Read the model definition and answer for the solid it produces. Units are mm, in the model's axes. Face numbers are marked on the shaded views. A direction names the side the tool comes from. Round coordinates to 2 decimals unless told otherwise and drop trailing zeros. Order: outer loops, then holes, each group sorted by start corner. A loop starts at its lowest first (then second) coordinate and runs counter-clockwise, first axis right, second up. Notation, with made-up numbers: (41.5, 79) -> (81.5, 79) arc R21 cw to (81.5, 109) -> close; hole circle Ø6 at (33.5, -37). An arc over 180 degrees is marked (long way). Answer as a JSON object with one key per item and string values. Group by question number.
Item 1: The mould has two halves that part along Z. Classify the marked faces 1, 2, 3 and 4: pulls with the +Z half, pulls with the -Z half, needs draft (parallel to the pull), parting line crosses it, or undercut.
Item 2: Section D-D, the plane z = 30 is taken. Write down the section's boundary in (x, y).
Item 3: Section A-A, the plane z = 5.5 is taken. Write down the section's boundary in (x, y), plus the area to 3 significant figures.
Item 4: For the marked faces 5 and 6, determine the directions among +Z, -Z, +X, -X, +Y, -Y from which every point of the face is accessible in a straight line to the end or side of a thin tool.
Item 5: Given P1, Ø9, axis at x = -70, y = 5, coming from the +Z side; P2, Ø17, axis at x = -71.95, y = 0, coming from the -Z side; P3, Ø4, axis at y = -5, z = 26, coming from the +X side, each flat-ended and moving along its own axis, determine where each tip first touches the part or whether it passes through.
Item 6: Section C-C, the plane y = 4.25 is taken. Write down the section's boundary in (x, z).
Item 7: Section B-B, the plane x = 130 is taken. Write down the section's boundary in (y, z), plus the area to 3 significant figures.
Item 8: Consider probe 1 along X at (y, z) = (-1.5, -14.5); probe 2 along X at (y, z) = (-1.25, 15); probe 3 along X at (y, z) = (-8.75, -20.5). Determine where each line is inside the solid, lowest interval first. Write a range as from..to.
from build123d import *
from build123d.topology import SkipClean

# Parameters (mm, degrees)
SKETCH1_R           = 50
BOSS_EXTRUDE4_DEPTH = 10
SKETCH4_R           = 50
BOSS_EXTRUDE5_DEPTH = 5
BOSS_EXTRUDE6_START = 5
SKETCH5_R           = 50
BOSS_EXTRUDE6_DEPTH = 5
SKETCH9_R           = 15
SKETCH9_R_2         = 7.5
BOSS_EXTRUDE8_DEPTH = 40
CUT_EXTRUDE1_START  = 50
SKETCH11_R          = 15
CUT_EXTRUDE1_DEPTH  = 50
BOSS_EXTRUDE9_START = 12
SKETCH12_R          = 7.5
BOSS_EXTRUDE9_DEPTH = 12


with BuildPart() as part:
    # Sketch1 → Boss-Extrude4 (new, symmetric)
    # profile 1 of 2: a face of its own
    with BuildSketch(Plane(origin=(0, 0, 0), x_dir=(1, 0, 0), z_dir=(0, 1, 0))):
        with BuildLine():
            Line((109.631487436, 59.370873009), (-60.952961118, 36.317806))
            Line((-60.952961118, 36.317806), (-60.952961118, -47.492515538))
            Line((-60.952961118, -47.492515538), (113.395395748, -59.936377162))
            ThreePointArc((113.395395748, -59.936377162), (57.696778774, -1.980561591), (109.631487436, 59.370873009))
        make_face()
        with BuildLine():
            Line((-46.622582391, 28.163534109), (48.543183, 41.024394434))
            ThreePointArc((48.543183, 41.024394434), (53.334657365, 38.899688702), (53.596610708, 33.664807473))
            ThreePointArc((53.596610708, 33.664807473), (45.011329084, -2.407953952), (56.056582269, -37.805038006))
            ThreePointArc((56.056582269, -37.805038006), (56.147884391, -43.057885165), (51.492525841, -45.492710855))
            Line((51.492525841, -45.492710855), (-46.308923365, -38.512273973))
            ThreePointArc((-46.308923365, -38.512273973), (-49.612183114, -36.932319839), (-50.952961118, -33.524960981))
            Line((-50.952961118, -33.524960981), (-50.952961118, 23.208576253))
            ThreePointArc((-50.952961118, 23.208576253), (-49.717805495, 26.498856913), (-46.622582391, 28.163534109))
        make_face(mode=Mode.SUBTRACT)
    # profile 2 of 2: a face of its own
    with BuildSketch(Plane(origin=(0, 0, 0), x_dir=(1, 0, 0), z_dir=(0, 1, 0))):
        with BuildLine():
            ThreePointArc((177.666942704, -0.088621259), (157.15031062, 45.089511261), (109.631487436, 59.370873009))
            ThreePointArc((109.631487436, 59.370873009), (57.696778774, -1.980561591), (113.395395748, -59.936377162))
            ThreePointArc((113.395395748, -59.936377162), (158.555248995, -43.999285211), (177.666942704, -0.088621259))
        make_face()
        with Locations(Location((117.666942704, -0.088621259, 0), (0, 0, 270))):
            Circle(SKETCH1_R, mode=Mode.SUBTRACT)
    extrude(amount=BOSS_EXTRUDE4_DEPTH, both=True)

    # Sketch4 → Boss-Extrude5 (add)
    with BuildSketch(Plane(origin=(0, 10, 0), x_dir=(1, 0, 0), z_dir=(0, 1, 0))):
        with BuildLine():
            ThreePointArc((109.631487436, 59.370873009), (57.696778774, -1.980561591), (113.395395748, -59.936377162))
            ThreePointArc((113.395395748, -59.936377162), (158.555248995, -43.999285211), (177.666942704, -0.088621259))
            ThreePointArc((177.666942704, -0.088621259), (157.15031062, 45.089511261), (109.631487436, 59.370873009))
        make_face()
        with Locations(Location((117.666942704, -0.088621259, 0), (0, 0, 270))):
            Circle(SKETCH4_R, mode=Mode.SUBTRACT)
    extrude(amount=BOSS_EXTRUDE5_DEPTH)

    # Sketch5 → Boss-Extrude6 (add)
    with BuildSketch(Plane.XZ.offset(10).offset(BOSS_EXTRUDE6_START)):
        with BuildLine():
            ThreePointArc((113.395395748, 59.936377162), (57.696778774, 1.980561591), (109.631487436, -59.370873009))
            ThreePointArc((109.631487436, -59.370873009), (157.15031062, -45.089511261), (177.666942704, 0.088621259))
            ThreePointArc((177.666942704, 0.088621259), (158.555248995, 43.999285211), (113.395395748, 59.936377162))
        make_face()
        with Locations(Location((117.666942704, 0.088621259, 0), (0, 0, 270))):
            Circle(SKETCH5_R, mode=Mode.SUBTRACT)
    extrude(amount=-BOSS_EXTRUDE6_DEPTH)

    # Sketch9 → Boss-Extrude8 (add, symmetric)
    with SkipClean():  # the faces are left unmerged after this step: merging them gives an invalid solid
        with BuildSketch(Plane.XY):
            with Locations(Location((-71.952961118, 0, 0), (0, 0, 318.189685104))):
                Circle(SKETCH9_R)
            with Locations((-71.952961118, 0)):
                Circle(SKETCH9_R_2, mode=Mode.SUBTRACT)
        extrude(amount=BOSS_EXTRUDE8_DEPTH, both=True)

    # Sketch11 → Cut-Extrude1 (cut)
    with SkipClean():  # the faces are left unmerged after this step: merging them gives an invalid solid
        with BuildSketch(Plane.XY.offset(40).offset(CUT_EXTRUDE1_START)):
            with Locations(Location((-71.952961118, 0, 0), (0, 0, 318.189685104))):
                Circle(SKETCH11_R)
        extrude(amount=-CUT_EXTRUDE1_DEPTH, mode=Mode.SUBTRACT)

    # Sketch12 → Boss-Extrude9 (add)
    with SkipClean():  # the faces are left unmerged after this step: merging them gives an invalid solid
        with BuildSketch(Plane.XY.offset(40).offset(BOSS_EXTRUDE9_START)):
            with BuildLine():
                ThreePointArc((-60.772621231, 10), (-86.952961118, 0), (-60.772621231, -10))
                ThreePointArc((-60.772621231, -10), (-56.952961118, 0), (-60.772621231, 10))
            make_face()
            with Locations((-71.952961118, 0)):
                Circle(SKETCH12_R, mode=Mode.SUBTRACT)
        extrude(amount=-BOSS_EXTRUDE9_DEPTH)


solid = part.part
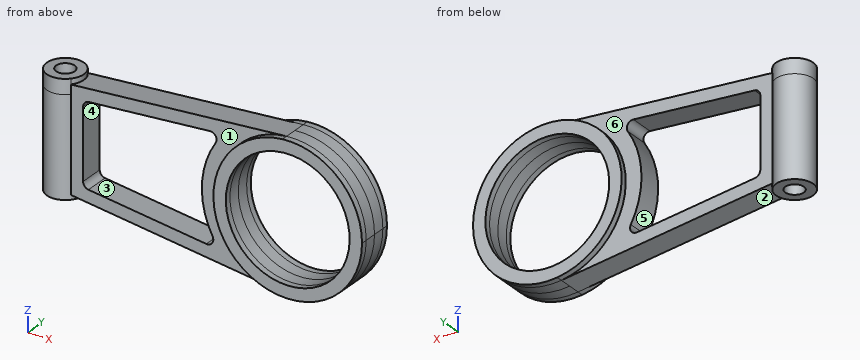
Values found:
{
 "1": {"face 1": "needs draft", "face 2": "pulls with the -Z half", "face 3": "undercut", "face 4": "undercut"},
 "2": {"outline": "(-60.77, -10) -> (-50.95, -10) -> (-50.95, 10) -> (-60.77, 10) arc R15 ccw (long way) to start; (51.72, -10) -> (65.65, -10) -> (65.65, -15) -> (77.6, -15) -> (77.6, 15) -> (65.65, 15) -> (65.65, 10) -> (51.72, 10) -> close; (157.73, -15) -> (169.68, -15) -> (169.68, 15) -> (157.73, 15) -> close; hole circle Ø15 at (-71.95, 0)"},
 "3": {"outline": "(-60.77, -10) -> (-50.95, -10) -> (-50.95, 10) -> (-60.77, 10) arc R15 ccw (long way) to start; (45.19, -10) -> (57.91, -10) -> (57.91, -15) -> (67.96, -15) -> (67.96, 15) -> (57.91, 15) -> (57.91, 10) -> (45.19, 10) -> close; (167.37, -15) -> (177.42, -15) -> (177.42, 15) -> (167.37, 15) -> close; hole circle Ø15 at (-71.95, 0)", "area": "1,530 mm2"},
 "4": {"face 5": "+Y, -Y", "face 6": "+Y"},
 "5": {"P1": "z = 52", "P2": "z = -40", "P3": "x = 172.7"},
 "6": {"outline": "(-86.34, -40) -> (-78.13, -40) -> (-78.13, 52) -> (-86.34, 52) -> close; (-65.77, -40) -> (-57.57, -40) -> (-57.57, -36.78) -> (109.63, -59.37) arc R60 ccw (long way) to (113.4, 59.94) -> (-57.57, 47.73) -> (-57.57, 52) -> (-65.77, 52) -> close; hole (-50.95, -23.21) arc R5 ccw to (-46.62, -28.16) -> (48.54, -41.02) arc R5 ccw to (53.6, -33.66) arc R70 cw to (56.06, 37.81) arc R5 ccw to (51.49, 45.49) -> (-46.31, 38.51) arc R5 ccw to (-50.95, 33.52) -> close; hole circle Ø100 at (117.67, 0.09)"},
 "7": {"outline": "(-15, -58.63) -> (15, -58.63) -> (15, -48.37) -> (-15, -48.37) -> close; (-15, 48.54) -> (15, 48.54) -> (15, 58.81) -> (-15, 58.81) -> close", "area": "616 mm2"},
 "8": {"probe 1": "-86.88..-79.3, -64.6..-50.95, 46.49..69.84, 165.49..175.87", "probe 2": "-86.9..-79.35, -64.56..-50.95, 46.6..69.94, 165.39..175.78", "probe 3": "-84.14..-50.95, 48.04..72.1, 163.23..174.02"}
}
